from build123d import *

# Parameters (mm, degrees)
F0_W     = 132.177695632
F0_H     = 127.1953880787
F1_DEPTH = 82.296
F2_R     = 10.4245741623
F3_R     = 13.4906253865
F4_T     = -2.54


# Not quite as in the source:
# - a shell that OpenCascade refuses in one call is made with other operations: the cavity is built on its own and cut out


with BuildPart() as f1:
    # F0 (on Front) → F1 (new body)
    with BuildSketch(Plane.XZ):
        with Locations((2.9307678342, -2.1980777383)):
            Rectangle(F0_W, F0_H)
    extrude(amount=F1_DEPTH)

    # F2
    f2_edges = [f1.edges().sort_by_distance(p)[0] for p in [
        (2.930768, -82.296, 61.399616),
        (-63.15808, -82.296, -2.198078),
        (2.930768, -82.296, -65.795772),
        (69.019616, -82.296, -2.198078),
    ]]
    fillet(f2_edges, radius=F2_R)

    # F3
    f3_edges = [f1.edges().sort_by_distance(p)[0] for p in [
        (2.930768, 0, 61.399616),
        (-63.15808, 0, -2.198078),
        (2.930768, 0, -65.795772),
        (69.019616, 0, -2.198078),
    ]]
    fillet(f3_edges, radius=F3_R)

    # F4: a shell. OpenCascade refuses it in one call, so the cavity is built on its own and cut out:
    # the body offset inwards by the wall thickness, plus a prism from it out through each open face.
    f4_core = offset(f1.part, amount=F4_T, mode=Mode.PRIVATE)
    f4_exits = [f4_core.faces().sort_by_distance(p)[0] for p in [
        (2.930768, -79.756, -2.198078),
        (2.930768, -2.54, -2.198078),
    ]]
    add(f4_core, mode=Mode.SUBTRACT)
    extrude(f4_exits, amount=-F4_T, mode=Mode.SUBTRACT)


solid = f1.part
Read the model definition and answer for the solid it produces. Units are mm, in the model's axes. A direction names the side the tool comes from. Give positions to 0.01 mm unless a question says otherwise; leave off trailing zeros. Loops run counter-clockwise (first coordinate to the right, second up) from the corner with the lowest first, then second, coordinate; pieces in that order, holes last. Notation, with made-up numbers: (-37.75, 18) - (-1.75, 18) arc R20 cw to (-1.75, 23) - close; hole circle Ø10 at (80.25, 79.5). An arc over 180 degrees is marked (long way). Answer as CSV lines item,"result". Start each with the question number.
1) Find section B-B (z = -41). Write down the section's boundary in (x, y), then the cut area to 3 significant figures.
2) Which of the six approach directions +Z, -Z, +X, -X, +Y, -Y give full straight-line access (tool end or side, diameter ignored) to faces 1 (the face through (-59.311, -4.057, -1.308)), 2 (the face through (-58.37, -77.385, -1.343))?
3) Straight lines are drawn through the part: L1, parallel to Z at x = -56.5, y = -32.5; L2, parallel to X at y = -62.5, z = 14; L3, parallel to X at y = -11, z = 47.5. For each, find the intervals that lie inside material, in ascending order. Write a range as from..to.
4) Each of these flat-tipped pins is pushed along its axis until it touches: pin 1 Ø2 at (y, z) = (-1.5, -4.5) entering from -X; pin 2 Ø1.3 at (x, y) = (27.5, -1) entering from +Z; pin 3 Ø3 at (x, y) = (9, -0.5) entering from -Z; pin 4 Ø1 at (x, z) = (41.5, -50) entering from +Y. Where does it stop, or does it pass through?
5) Find section A-A (x = -27.5). Write down the section's boundary in (y, z).
6) Find section C-C (y = -33.5). Write down the section's boundary in (x, z), then the cut area to 3 significant figures.
7) Determine the mould class of faces 3 (the face through (2, -42, -65.796)), 4 (the face through (64.963, -3.847, -1.308)), 5 (the face through (-63.158, -42, -3)), 6 (the face through (64.231, -77.385, -1.343)) for opening direction X: released by +X, released by -X, zero draft, split by the parting line, or undercut.
8) Find section D-D (z = 53.5). Write down the section's boundary in (x, y), then the cut area to 3 significant figures.
Findings below:
1,outline,"(-63.16, -71.87) arc R10.42 ccw to (-52.73, -82.3) - (-52.73, -79.76) arc R7.88 cw to (-60.62, -71.87) - (-60.62, -13.49) arc R10.95 cw to (-49.67, -2.54) - (-49.67, 0) arc R13.49 ccw to (-63.16, -13.49) - close; (55.53, -2.54) arc R10.95 cw to (66.48, -13.49) - (66.48, -71.87) arc R7.88 cw to (58.6, -79.76) - (58.6, -82.3) arc R10.42 ccw to (69.02, -71.87) - (69.02, -13.49) arc R13.49 ccw to (55.53, 0) - close"
1,area,"467 mm^2"
2,face 1,"+Z, -Z, -X, +Y"
2,face 2,"none"
3,L1,"-65.8..-63.26, 58.86..61.4"
3,L2,"-63.16..-60.62, 66.48..69.02"
3,L3,"-62.93..-60.33, 66.19..68.79"
4,pin 1,"x = -57.49"
4,pin 2,"z = 54.37"
4,pin 3,"z = -59.37"
4,pin 4,"through"
5,outline,"(-82.3, -55.37) arc R10.42 ccw to (-71.87, -65.8) - (-13.49, -65.8) arc R13.49 ccw to (0, -52.31) - (-2.54, -52.31) arc R10.95 cw to (-13.49, -63.26) - (-71.87, -63.26) arc R7.88 cw to (-79.76, -55.37) - close; (-82.3, 50.98) - (-79.76, 50.98) arc R7.88 cw to (-71.87, 58.86) - (-13.49, 58.86) arc R10.95 cw to (-2.54, 47.91) - (0, 47.91) arc R13.49 ccw to (-13.49, 61.4) - (-71.87, 61.4) arc R10.42 ccw to start"
6,outline,"(-63.16, -65.8) - (69.02, -65.8) - (69.02, 61.4) - (-63.16, 61.4) - close; hole (-60.62, -63.26) - (66.48, -63.26) - (66.48, 58.86) - (-60.62, 58.86) - close"
6,area,"1,290 mm^2"
7,face 3,"zero draft"
7,face 4,"released by +X"
7,face 5,"released by -X"
7,face 6,"undercut"
8,outline,"(-63.16, -71.87) arc R10.42 ccw to (-55.26, -81.99) - (61.12, -81.99) arc R10.42 ccw to (69.02, -71.87) - (69.02, -13.49) arc R13.49 ccw to (61.12, -1.21) - (-55.26, -1.21) arc R13.49 ccw to (-63.16, -13.49) - close; hole (-60.62, -71.87) arc R7.88 ccw to (-55.26, -79.34) - (61.12, -79.34) arc R7.88 ccw to (66.48, -71.87) - (66.48, -13.49) arc R10.95 ccw to (61.12, -4.07) - (-55.26, -4.07) arc R10.95 ccw to (-60.62, -13.49) - close"
8,area,"1,070 mm^2"
